Autodesk Inventor part; units mm, degrees
ref_plane "YZ Plane" through (0, 0, 0) normal (1, 0, 0) x (0, 1, 0)
ref_plane "XZ Plane" through (0, 0, 0) normal (0, 1, 0) x (-1, 0, 0)
ref_plane "XY Plane" through (0, 0, 0) normal (0, 0, 1) x (1, 0, 0)
sketch "Sketch1" plane through (0, 0, 0) normal (0, 1, 0) x (-1, 0, 0)
  line L0 (5, 5) -> (-5, 5)
  line L1 (-5, 5) -> (-5, -5)
  line L2 (-5, -5) -> (5, -5)
  line L3 (5, -5) -> (5, 5)
  line L4 (5, 5) -> (-5, -5) construction
  line L5 (-5, 5) -> (5, -5) construction
  circle A0 centre (0, 9) radius 2.25
  line L6 (5, 0) -> (7.8618, 0)
  circle A1 centre (0, -9) radius 2.25
  line L7 (5, -9) -> (5, -5)
  line L8 (-5, -9) -> (-5, -5)
  line L9 (-5, 5) -> (5, 5)
  line L10 (5, 5) -> (5, 13)
  line L11 (5, 13) -> (-5, 13)
  line L12 (-5, 13) -> (-5, 5)
  line L13 (-5, -5) -> (5, -5)
  line L14 (5, -5) -> (5, -13)
  line L15 (5, -13) -> (-5, -13)
  line L16 (-5, -13) -> (-5, -5)
  point P0 (0, 0)
  dimension "d0" = 10
  dimension "d1" = 10
  dimension "d2" = 4.5
  dimension "d4" = 4
  dimension "d17" = 4
extrude "Extrusion1" add sketch "Sketch1" along normal blind 3
sketch "Sketch2" plane through (0, 3, 0) normal (0, 1, 0) x (1, 0, 0)
  line L0 (-5, 5) -> (-5, -5)
  line L1 (5, -5) -> (-5, -5)
  line L2 (-5, -5) -> (-5, 5)
  line L3 (-5, 5) -> (5, 5)
  line L4 (5, 5) -> (5, -5)
  line L5 (5, -5) -> (-5, 5) construction
  line L6 (-5, -5) -> (5, 5) construction
  point P0 (0, 0)
  point P1 (-5, 9)
  point P2 (-5, -9)
  dimension "d8" = 10
extrude "Extrusion2" add sketch "Sketch2" along normal blind 82
mirror "Mirror1" about plane through (0, 85, 0) normal (0, 1, 0) of "Extrusion1", "Extrusion2"
properties part number "basket_pilar"
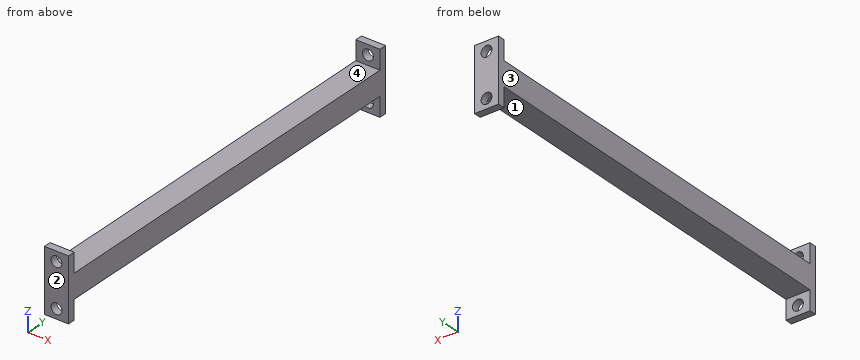
Input: part model. Units: mm. Frame: model coordinates. Face numbers are marked on the shaded views. Coordinates: 2 decimals unless noted, no trailing zeros. Write each loop counter-clockwise with the first axis right and the second up, starting at its lowest first coordinate (ties: lowest second). Pieces come first, ordered by that corner, then holes. Notation, with made-up numbers: (50.5, 74.25) -> (63.5, 74.25) arc R17 cw to (63.5, 103.25) -> close; hole circle Ø5 at (41.5, -39.5). An arc over 180 degrees is marked (long way). Answer as a JSON object with one key per item and string values.
1. Section A-A on z = 9. Return the cut outline in (x, y).
Result set:
{"outline": "(-5, 0) -> (-2.25, 0) -> (-2.25, 3) -> (-5, 3) -> close; (-5, 167) -> (-2.25, 167) -> (-2.25, 170) -> (-5, 170) -> close; (2.25, 0) -> (5, 0) -> (5, 3) -> (2.25, 3) -> close; (2.25, 167) -> (5, 167) -> (5, 170) -> (2.25, 170) -> close"}
2. First-contact query: P1, Ø1.5, axis at x = -3.5, y = 25.5, coming from the -Z side; P2, Ø2, axis at x = -2.5, y = 29.5, coming from the +Z side. Flat tips, straight axial feed; report the tip coordinate or a pass-through.
Result set:
{"P1": "stops at z = -5", "P2": "stops at z = 5"}
3. Section B-B on x = 0.25. Return the cut outline in (y, z), then the cut area to 3 significant figures.
Result set:
{"outline": "(0, -13) -> (3, -13) -> (3, -11.24) -> (0, -11.24) -> close; (0, -6.76) -> (3, -6.76) -> (3, -5) -> (167, -5) -> (167, -6.76) -> (170, -6.76) -> (170, 6.76) -> (167, 6.76) -> (167, 5) -> (3, 5) -> (3, 6.76) -> (0, 6.76) -> close; (0, 11.24) -> (3, 11.24) -> (3, 13) -> (0, 13) -> close; (167, -13) -> (170, -13) -> (170, -11.24) -> (167, -11.24) -> close; (167, 11.24) -> (170, 11.24) -> (170, 13) -> (167, 13) -> close", "area": "1,740 mm2"}
4. Mould query, pull axis Y, two halves, no side actions, for the marked faces 1, 2, 3 and 4. Classes: released by +Y, released by -Y, zero draft, split by the parting line, or undercut.
Result set:
{"face 1": "undercut", "face 2": "released by -Y", "face 3": "zero draft", "face 4": "undercut"}
5. Material intervals for line 1 (Z direction, x = 0, y = 0.85); line 2 (Y direction, x = 4.5, z = -11.25); line 3 (Z direction, x = -1.5, y = 63), sorted ascending. Write a range as from..to.
Result set:
{"line 1": "z = -13..-11.25, -6.75..6.75, 11.25..13", "line 2": "y = 0..3, 167..170", "line 3": "z = -5..5"}
6. Section C-C on y = 23. Return the cut outline in (x, z), then the cut area to 3 significant figures.
Result set:
{"outline": "(-5, -5) -> (5, -5) -> (5, 5) -> (-5, 5) -> close", "area": "100 mm2"}
